Read the model definition and answer for the solid it produces. Units are mm, in the model's axes. Face numbers are marked on the shaded views. A direction names the side the tool comes from. Round coordinates to 2 decimals unless told otherwise and drop trailing zeros. Order: outer loops, then holes, each group sorted by start corner. A loop starts at its lowest first (then second) coordinate and runs counter-clockwise, first axis right, second up.
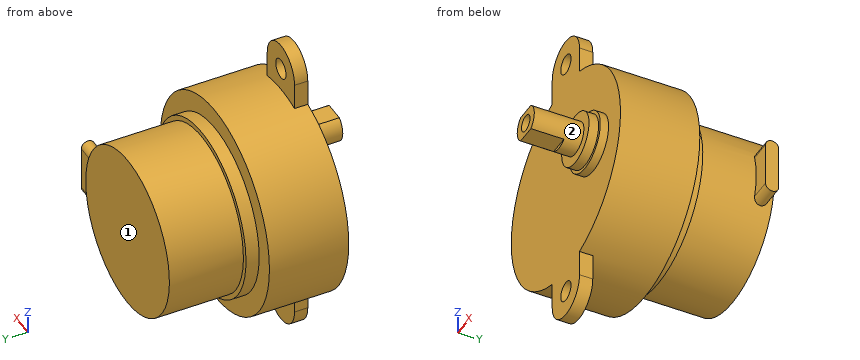
from build123d import *

# Parameters (mm, degrees)
SKETCH_9_W          = 5.698212476
SKETCH_9_H          = 1.620294685
SKETCH_9_W_2        = 7.400009417
SKETCH_9_H_2        = 3.482357373
CUT_EXTRUDE_1_DEPTH = 5
SKETCH_10_R         = 1.5
EXTRUDE_5_DEPTH     = 2
EXTRUDE_6_DEPTH     = 15


with BuildPart() as part:
    # Sketch 3 → Revolve 1 (revolve)
    with BuildSketch(Plane.XY, mode=Mode.PRIVATE) as revolve_1_sk:
        Polygon((-16, 0), (-16, 12), (-13, 12), (-13, 14), (-12.25, 14), (-12.25, 25.2), (0, 25.2), (0, 0), align=None)
    revolve(revolve_1_sk.sketch.rotate(Axis((0, 0, 0), (0, 1, 0)), 270), axis=Axis((0, 0, 0), (0, 1, 0)))



with BuildPart() as body_2:
    # Sketch 6 → Revolve 4 (revolve)
    with BuildSketch(Plane.XY):
        Polygon((3.5, 0), (3.5, -1.25), (4, -1.25), (4, -2.7), (5.5, -2.7), (5.5, -10.2), (8, -10.2), (8, -5.2), (8, 0), align=None)
    revolve(axis=Axis((8, 0, 0), (0, -1, 0)))

    # Sketch 8 → Hole Wizard M3 _1 (revolve, cut)
    with BuildSketch(Plane(origin=(8, -10.2, 0), x_dir=(0, 0, -1), z_dir=(1, 0, 0))):
        Polygon((0, 0), (0, 8.251075774), (1.25, 7.5), (1.25, 0), align=None)
    revolve(axis=Axis((8, -16.55, 0), (0, 1, 0)), mode=Mode.SUBTRACT)

    # Sketch 9 → Cut-Extrude 1 (cut)
    with BuildSketch(Plane.XZ.offset(10.2)):
        with Locations((8.176379841, 2.810147343)):
            Rectangle(SKETCH_9_W, SKETCH_9_H)
        with Locations((7.325481371, -3.741178687)):
            Rectangle(SKETCH_9_W_2, SKETCH_9_H_2)
    extrude(amount=-CUT_EXTRUDE_1_DEPTH, mode=Mode.SUBTRACT)


with BuildPart() as part_1:
    add(part.part)

    add(body_2.part)  # Extrude 5 merges body 2
    # Sketch 10 → Extrude 5 (add)
    with BuildSketch(Plane.XZ):
        with BuildLine():
            Line((-4, -19.5), (-4, 19.5))
            ThreePointArc((-4, 19.5), (0, 23.5), (4, 19.5))
            Line((4, 19.5), (4, -19.5))
            ThreePointArc((4, -19.5), (0, -23.5), (-4, -19.5))
        make_face()
        with Locations(Location((0, 19.5, 0), (0, 0, 270))):
            Circle(SKETCH_10_R, mode=Mode.SUBTRACT)
        with Locations(Location((0, -19.5, 0), (0, 0, 270))):
            Circle(SKETCH_10_R, mode=Mode.SUBTRACT)
    extrude(amount=-EXTRUDE_5_DEPTH)

    # Sketch 11 → Extrude 6 (add)
    with BuildSketch(Plane(origin=(0, 0, 0), x_dir=(0, 0, -1), z_dir=(1, 0, 0))):
        with BuildLine():
            Line((-3.311772074, 24.45726904), (3.311772074, 24.45726904))
            ThreePointArc((3.311772074, 24.45726904), (4.30779375, 23.461247363), (3.311772074, 22.465225687))
            Line((3.311772074, 22.465225687), (-3.311772074, 22.465225687))
            ThreePointArc((-3.311772074, 22.465225687), (-4.30779375, 23.461247363), (-3.311772074, 24.45726904))
        make_face()
    extrude(amount=EXTRUDE_6_DEPTH)


solid = part_1.part
Q1. Flat-ended cylindrical pins translate along their axes: pin 1 (1 mm diameter, centred on x = 8, z = -9.5, fed in from +Y); pin 2 (4 mm diameter, centred on x = -1.5, z = -21, fed in from +Y); pin 3 (12 mm diameter, centred on y = -4.5, z = -9.5, fed in from +X); pin 4 (1 mm diameter, centred on y = 10, z = 13.5, fed in from +X). Find the tip coordinate at first contact, or state that the pin passes through.
Outcome:
pin 1: stops at y = 25.2
pin 2: stops at y = 2
pin 3: stops at x = 15.01
pin 4: stops at x = 9.33
Q2. A cutting plane is placed at A-A, the plane x = 0. Give the vertices of the cut face in (y, z).
Outcome:
outline: (0, -23.5) - (2, -23.5) - (2, -21) - (0, -21) - close; (0, -18) - (2, -18) - (2, -16) - (12, -16) - (12, -13) - (14, -13) - (14, -12.25) - (25.2, -12.25) - (25.2, 12.25) - (14, 12.25) - (14, 13) - (12, 13) - (12, 16) - (2, 16) - (2, 18) - (0, 18) - close; (0, 21) - (2, 21) - (2, 23.5) - (0, 23.5) - close
Q3. A cutting plane is placed at D-D, the plane y = 10.5. Give the vertices of the cut face in (x, z), plus the area to 3 significant figures.
Outcome:
outline: circle Ø32 at (0, 0)
area: 804 mm2
Q4. A cutting plane is placed at C-C, the plane y = -4. Give the vertices of the cut face in (x, z), plus the area to 3 significant figures.
Outcome:
outline: circle Ø5 at (8, 0); hole circle Ø2.5 at (8, 0)
area: 14.7 mm2
Q5. For the marked faces 1 and 2, determine the directions among +Z, -Z, +X, -X, +Y, -Y from which every point of the face is accessible in a straight line to the end or side of a thin tool.
Outcome:
face 1: +Z, -Z, +X, -X, +Y
face 2: -Y
Q6. A cutting plane is placed at B-B, the plane z = -10. Give the vertices of the cut face in (x, y), plus the area to 3 significant figures.
Outcome:
outline: (-12.49, 0) - (12.49, 0) - (12.49, 12) - (8.31, 12) - (8.31, 14) - (7.08, 14) - (7.08, 25.2) - (-7.08, 25.2) - (-7.08, 14) - (-8.31, 14) - (-8.31, 12) - (-12.49, 12) - close
area: 491 mm2
Q7. Straight lines are drawn through the part: probe 1 along X at (y, z) = (1.05, -19.5); probe 2 along Z at (x, y) = (8, -5.5); probe 3 along Y at (x, z) = (-8, -7). For each, find the intervals that lie inside material, in ascending order.
Outcome:
probe 1: x = -4 to -1.5, 1.5 to 4
probe 2: z = -2 to -1.25, 1.25 to 2
probe 3: y = 0 to 25.2
